Can you work these out from the model? Positions are in its coordinate system, mm. Give positions to 0.01 mm unless a question says otherwise; leave off trailing zeros. Write each loop counter-clockwise with the first axis right and the second up, starting at its lowest first coordinate (ties: lowest second). Pieces come first, ordered by that corner, then holes. Notation, with made-up numbers: (-32, 69) - (-13, 69) arc R21 ccw to (-13, 95) - close; hole circle Ø9 at (78, 31). An arc over 180 degrees is marked (long way). Use a Markdown table: item, result. Add a question column.
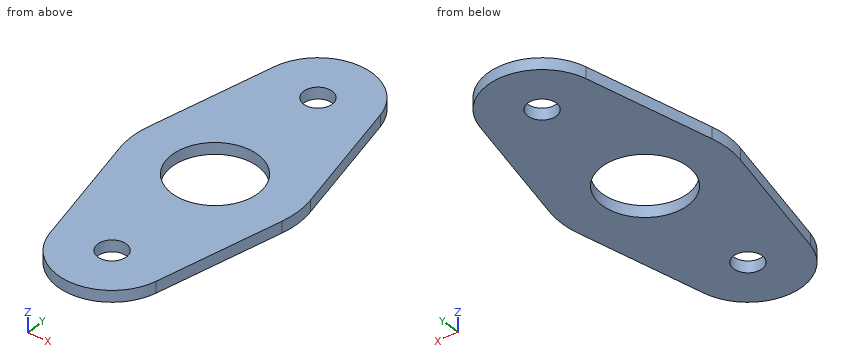
```python
from build123d import *

# Parameters (mm, degrees)
SKETCH1_R           = 7.5
SKETCH1_R_2         = 2.5
BOSS_EXTRUDE1_DEPTH = 1


with BuildPart() as part:
    # Sketch1 → Boss-Extrude1 (new, symmetric)
    with BuildSketch(Plane.XY):
        with BuildLine():
            Line((-9.272803089, 25.065217391), (-14.153225767, 3.152173913))
            ThreePointArc((-14.153225767, 3.152173913), (-14.5, 0), (-14.153225767, -3.152173913))
            Line((-14.153225767, -3.152173913), (-9.272803089, -25.065217391))
            ThreePointArc((-9.272803089, -25.065217391), (0, -32.5), (9.272803089, -25.065217391))
            Line((9.272803089, -25.065217391), (14.153225767, -3.152173913))
            ThreePointArc((14.153225767, -3.152173913), (14.5, 0), (14.153225767, 3.152173913))
            Line((14.153225767, 3.152173913), (9.272803089, 25.065217391))
            ThreePointArc((9.272803089, 25.065217391), (0, 32.5), (-9.272803089, 25.065217391))
        make_face()
        Circle(SKETCH1_R, mode=Mode.SUBTRACT)
        with Locations((0, 23)):
            Circle(SKETCH1_R_2, mode=Mode.SUBTRACT)
        with Locations(Location((0, -23, 0), (0, 0, 180))):
            Circle(SKETCH1_R_2, mode=Mode.SUBTRACT)
    extrude(amount=BOSS_EXTRUDE1_DEPTH, both=True)


solid = part.part
```
Q1. Suppose I cut it at D-D (y = 6.5). Please give me the cut outline in (x, z), and give its area (3 significant figures).
Q2. Suppose I cut it at A-A (y = 0). Please give me the cut outline in (x, z), and give its area (3 significant figures).
Q3. I'm going to push flat-ended pins straight in: P1, Ø3, axis at x = 0, y = 23, coming from the +Z side; P2, Ø1, axis at y = -7.5, z = 0.5, coming from the +X side. Where does each tip first touch, or does it pass through?
Q4. If I drill on probe 1 along Y at (x, z) = (0, -0.5); probe 2 along Y at (x, z) = (2, 0.7); probe 3 along X at (y, z) = (-3, 0.85), over which ranges is the centre line in solid material (lowest first)? Write a range as [from, to].
Q5. Suppose I cut it at C-C (x = 0). Please give me the cut outline in (y, z).
Q6. Suppose I cut it at B-B (z = -0.45). Please give me the cut outline in (x, y), and give its area (3 significant figures).
Derived:
| question | item | result |
|---|---|---|
| 1 | outline | (-13.41, -1) - (-3.74, -1) - (-3.74, 1) - (-13.41, 1) - close; (3.74, -1) - (13.41, -1) - (13.41, 1) - (3.74, 1) - close |
| 1 | area | 38.7 mm² |
| 2 | outline | (-14.5, -1) - (-7.5, -1) - (-7.5, 1) - (-14.5, 1) - close; (7.5, -1) - (14.5, -1) - (14.5, 1) - (7.5, 1) - close |
| 2 | area | 28.0 mm² |
| 3 | P1 | through |
| 3 | P2 | x = 13.3 |
| 4 | probe 1 | [-32.5, -25.5], [-20.5, -7.5], [7.5, 20.5], [25.5, 32.5] |
| 4 | probe 2 | [-32.29, -24.5], [-21.5, -7.23], [7.23, 21.5], [24.5, 32.29] |
| 4 | probe 3 | [-14.19, -6.87], [6.87, 14.19] |
| 5 | outline | (-32.5, -1) - (-25.5, -1) - (-25.5, 1) - (-32.5, 1) - close; (-20.5, -1) - (-7.5, -1) - (-7.5, 1) - (-20.5, 1) - close; (7.5, -1) - (20.5, -1) - (20.5, 1) - (7.5, 1) - close; (25.5, -1) - (32.5, -1) - (32.5, 1) - (25.5, 1) - close |
| 6 | outline | (-14.15, -3.15) - (-9.27, -25.07) arc R9.5 ccw to (9.27, -25.07) - (14.15, -3.15) arc R14.5 ccw to (14.15, 3.15) - (9.27, 25.07) arc R9.5 ccw to (-9.27, 25.07) - (-14.15, 3.15) arc R14.5 ccw to start; hole circle Ø15 at (0, 0); hole circle Ø5 at (0, -23); hole circle Ø5 at (0, 23) |
| 6 | area | 1,200 mm² |
